```python
from build123d import *

# Parameters (mm, degrees)
BOX020_W          = 71.8
BOX020_H          = 12
BOX020_DEPTH      = 9.5
CYLINDER024_R     = 7.9
CYLINDER024_DEPTH = 1.7
BOX002_W          = 32.25
BOX002_H          = 11
BOX002_DEPTH      = 30.25
CHAMFER_SIZE2     = 15
CHAMFER_SIZE      = 5
CHAMFER001_SIZE   = 5
CHAMFER002_SIZE   = 5
CHAMFER003_SIZE   = 10
CHAMFER004_SIZE   = 10
CHAMFER005_SIZE   = 10
CHAMFER006_SIZE   = 5
CHAMFER007_SIZE   = 1
CHAMFER008_SIZE   = 10


with BuildPart() as obj1:
    # Box020 → Box020 (new body)
    with BuildSketch(Plane(origin=(-40, 36.6, 10.375), x_dir=(1, 0, 0), z_dir=(0, 0, 1))):
        with Locations((35.9, 6)):
            Rectangle(BOX020_W, BOX020_H)
    extrude(amount=BOX020_DEPTH)


with BuildPart() as obj2:
    # Cylinder024 → Cylinder024 (new body)
    with BuildSketch(Plane(origin=(30.1, 36.6, 15.125), x_dir=(0, 0, -1), z_dir=(1, 0, 0))):
        Circle(CYLINDER024_R)
    extrude(amount=CYLINDER024_DEPTH)

    # Cut001: cut obj1
    add(obj1.part, mode=Mode.SUBTRACT)


with BuildPart() as plunger_support:
    # Cone002 → Cone002 (revolve)
    with BuildSketch(Plane(origin=(33.5, 36.6, 15.125), x_dir=(0, 0, -1), z_dir=(0, -1, 0))):
        Polygon((0, 0), (7.9, 0), (0, 10), align=None)
    revolve(axis=Axis((33.5, 36.6, 15.125), (1, 0, 0)))


with BuildPart() as fusion009:
    # Box002 → Box002 (new body)
    with BuildSketch(Plane(origin=(26.25, 26.6, 0), x_dir=(1, 0, 0), z_dir=(0, 0, 1))):
        with Locations((16.125, 5.5)):
            Rectangle(BOX002_W, BOX002_H)
    extrude(amount=BOX002_DEPTH)

    # Chamfer
    chamfer_edges = [fusion009.edges().sort_by_distance(p)[0] for p in [
        (58.5, 37.6, 15.125),
    ]]
    chamfer_side = fusion009.faces().sort_by_distance((58.5, 32.1, 15.125))[0]
    chamfer(chamfer_edges, length=CHAMFER_SIZE, length2=CHAMFER_SIZE2, reference=chamfer_side)

    # Chamfer001
    chamfer001_edges = [fusion009.edges().sort_by_distance(p)[0] for p in [
        (34.875, 37.6, 30.25),
    ]]
    chamfer(chamfer001_edges, length=CHAMFER001_SIZE)

    # Chamfer002
    chamfer002_edges = [fusion009.edges().sort_by_distance(p)[0] for p in [
        (34.875, 37.6, 0),
    ]]
    chamfer(chamfer002_edges, length=CHAMFER002_SIZE)

    # Chamfer003
    chamfer003_edges = [fusion009.edges().sort_by_distance(p)[0] for p in [
        (26.25, 29.6, 0),
        (26.25, 29.6, 30.25),
    ]]
    chamfer(chamfer003_edges, length=CHAMFER003_SIZE)

    # Chamfer004
    chamfer004_edges = [fusion009.edges().sort_by_distance(p)[0] for p in [
        (36.25, 29.6, 0),
        (36.25, 29.6, 30.25),
    ]]
    chamfer(chamfer004_edges, length=CHAMFER004_SIZE)

    # Chamfer005
    chamfer005_edges = [fusion009.edges().sort_by_distance(p)[0] for p in [
        (46.25, 29.6, 30.25),
        (46.25, 29.6, 0),
    ]]
    chamfer(chamfer005_edges, length=CHAMFER005_SIZE)

    # Chamfer006
    chamfer006_edges = [fusion009.edges().sort_by_distance(p)[0] for p in [
        (43.5, 37.6, 15.125),
    ]]
    chamfer(chamfer006_edges, length=CHAMFER006_SIZE)

    # Chamfer007
    chamfer007_edges = [fusion009.edges().sort_by_distance(p)[0] for p in [
        (38.5, 37.6, 15.125),
    ]]
    chamfer(chamfer007_edges, length=CHAMFER007_SIZE)

    # Chamfer008
    chamfer008_edges = [fusion009.edges().sort_by_distance(p)[0] for p in [
        (48.243416, 36.018861, 15.125),
    ]]
    chamfer(chamfer008_edges, length=CHAMFER008_SIZE)

    # Fusion008: union plunger_support
    add(plunger_support.part)

    # Fusion009: union obj2
    add(obj2.part)


solid = fusion009.part
```
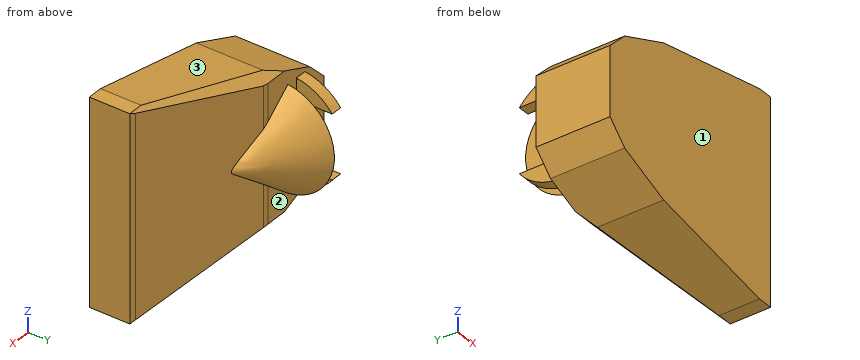
The model under review builds one solid part; all positions refer to its coordinate system, in mm. Face numbers are marked on the shaded views. Coordinates: 2 decimals unless noted, no trailing zeros. Loops run counter-clockwise (first coordinate to the right, second up) from the corner with the lowest first, then second, coordinate; pieces in that order, holes last. Notation, with made-up numbers: (34.5, -20.5) -> (64.5, -20.5) arc R26 cw to (64.5, 5.5) -> close; hole circle Ø1 at (-13, 67). An arc over 180 degrees is marked (long way). Answer as CSV lines item,"result".
Item 1: Insertion check: pin 1 (1.9 mm diameter, centred on x = 31, y = 39.5, fed in from -Z); pin 2 (0.9 mm diameter, centred on y = 39.5, z = 8, fed in from -X); pin 3 (5 mm diameter, centred on x = 34.5, y = 40.5, fed in from -Z). Each pin has a flat end and moves straight along its axis. Give the tip position at first contact, or say it passes through.
Results below:
pin 1,"stops at z = 7.47"
pin 2,"stops at x = 30.1"
pin 3,"stops at z = 7.39"
Item 2: Take a section at A-A, the plane y = 31.5. State the section outline as (x, z) points, and give its area (3 significant figures).
Results below:
outline,"(26.25, 10) -> (29.18, 7.07) -> (37.01, 3.83) -> (56.25, 0) -> (58.5, 0) -> (58.5, 30.25) -> (56.25, 30.25) -> (37.01, 26.42) -> (29.18, 23.18) -> (26.25, 20.25) -> close"
area,"767 mm2"
Item 3: Take a section at B-B, the plane y = 41.25. Count the separate pieces of the cut face and the enclosed holes in it, and give its area (3 significant figures).
Results below:
separate pieces,"3"
enclosed holes,"0"
area,"38.7 mm2"
Item 4: Draft analysis for pull direction Z (two halves, no side actions). For the marked faces 1, 2 and 3, state which applies: +Z half, -Z half, draft (parallel to the pull), parting line (faces both ways), or undercut.
Results below:
face 1,"draft"
face 2,"undercut"
face 3,"+Z half"
Item 5: For L1, parallel to Y at x = 30, z = 7; L2, parallel to Y at x = 55, z = 13; L3, parallel to Z at x = 33, y = 37, list the stretches that pass through material, from the lowest coordinate up.
Results below:
L1,"y = 26.6 to 37.6"
L2,"y = 26.6 to 33.52"
L3,"z = 5.49 to 24.76"
